from build123d import *

# Parameters (mm, degrees)
F0_R     = 9
F1_DEPTH = 3
F2_R     = 5.5
F3_DEPTH = 1
F4_R     = 1.25
F5_DEPTH = 9
F6_W     = 1.1
F6_H     = 3.75
F6_H_2   = 2.5
F7_DEPTH = 4.001


# Not quite as in the source:
# - a feature names something its author has since deleted; it is built from what else it names


with BuildPart() as f1:
    # F0 (on Top) → F1 (new body)
    with BuildSketch(Plane.XY):
        Circle(F0_R)
    extrude(amount=-F1_DEPTH)

    # F2 (on face) → F3 (join)
    with BuildSketch(Plane(origin=(0, 0, -3), x_dir=(1, 0, 0), z_dir=(0, 0, -1))):
        Circle(F2_R)
    extrude(amount=F3_DEPTH)

    # F4 (on Right) → F5 (cut, symmetric)
    with BuildSketch(Plane.YZ):
        Circle(F4_R)
    extrude(amount=F5_DEPTH, both=True, mode=Mode.SUBTRACT)

    # F6 (on face) → F7 (cut, through all)
    with BuildSketch(Plane.XY):
        with Locations((0, -3.125)):
            Rectangle(F6_W, F6_H)
        Rectangle(F6_W, F6_H_2)
        with Locations((0, 3.125)):
            Rectangle(F6_W, F6_H)
    extrude(amount=-F7_DEPTH, mode=Mode.SUBTRACT)


solid = f1.part
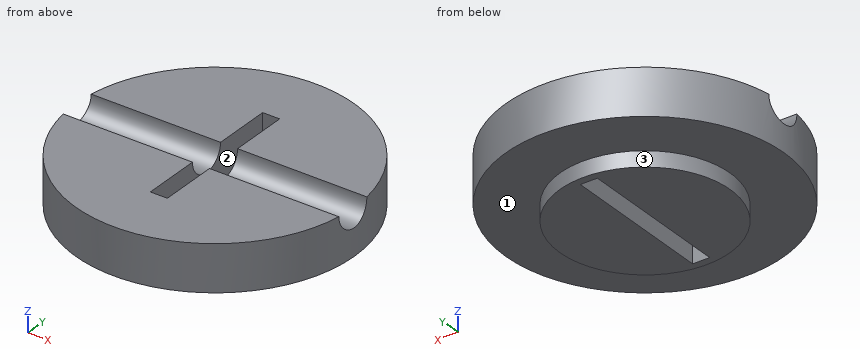
Input: part model. Units: mm. Frame: model coordinates. Face numbers are marked on the shaded views. Give positions to 0.01 mm unless a question says otherwise; leave off trailing zeros. Order: outer loops, then holes, each group sorted by start corner. A loop starts at its lowest first (then second) coordinate and runs counter-clockwise, first axis right, second up. Notation, with made-up numbers: M 38,-24.5 L 64,-24.5 A23 cw 64,10.5 Z; hole C 18,-33 d7. An arc over 180 degrees is marked long. Answer as a JSON object with one key per item and string values.
1. First-contact query: P1, Ø1.2, axis at y = -1.5, z = -2, coming from the +X side; P2, Ø1.2, axis at y = 2, z = -2.5, coming from the -X side. Flat tips, straight axial feed; report the tip coordinate or a pass-through.
Result sheet:
{"P1": "x = 8.95", "P2": "x = -8.89"}
2. Cut plane D-D, the plane x = -2.5. Output: boundary loops of the cut face in (y, z).
Result sheet:
{"outline": "M -8.65,-3 L -4.9,-3 L -4.9,-4 L 4.9,-4 L 4.9,-3 L 8.65,-3 L 8.65,0 L 1.25,0 A1.25 cw -1.25,0 L -8.65,0 Z"}
3. Cut plane C-C, the plane z = -0.45. Output: boundary loops of the cut face in (x, y), and give its area (3 significant figures).
Result sheet:
{"outline": "M -8.92,-1.17 A9 ccw 8.92,-1.17 L 0.55,-1.17 L 0.55,-5 L -0.55,-5 L -0.55,-1.17 Z; M -8.92,1.17 L -0.55,1.17 L -0.55,5 L 0.55,5 L 0.55,1.17 L 8.92,1.17 A9 ccw Z", "area": "204 mm²"}
4. Ray query, line 1 (X direction, y = 1.25, z = -1.5); line 2 (Y direction, x = -0.25, z = -2.1); line 3 (X direction, y = 2.75, z = -2.35). Return the intervals inside material, ascending. Write a range as [from, to].
Result sheet:
{"line 1": "[-8.91, -0.55], [0.55, 8.91]", "line 2": "[-9, -5], [5, 9]", "line 3": "[-8.57, -0.55], [0.55, 8.57]"}
5. Cut plane A-A, the plane x = 0. Output: boundary loops of the cut face in (y, z).
Result sheet:
{"outline": "M -9,-3 L -5.5,-3 L -5.5,-4 L -5,-4 L -5,0 L -9,0 Z; M 5,-4 L 5.5,-4 L 5.5,-3 L 9,-3 L 9,0 L 5,0 Z"}
6. Cut plane B-B, the plane z = -1.7. Output: boundary loops of the cut face in (x, y).
Result sheet:
{"outline": "C 0,0 d18; hole M -0.55,-5 L 0.55,-5 L 0.55,5 L -0.55,5 Z"}
7. Pull-direction query (X, two-part tool) for the marked faces 1, 2 and 3; classes: +X half, -X half, draft (parallel to the pull), parting line (faces both ways), or undercut.
Result sheet:
{"face 1": "draft", "face 2": "undercut", "face 3": "parting line"}
